Part model, mm, in its own coordinate system. Face numbers are marked on the shaded views. A direction names the side the tool comes from. Coordinates: 2 decimals unless noted, no trailing zeros. Loops run counter-clockwise (first coordinate to the right, second up) from the corner with the lowest first, then second, coordinate; pieces in that order, holes last.
```python
from build123d import *

# Parameters (mm, degrees)
BASPROSKE_W     = 20
BASPROSKE_H     = 48
TOOTHCUT_DEPTH  = 71.767224052
TEETHCUTS_COUNT = 22
TEETHCUTS_ANGLE = 343.636363636
BORSKE_R        = 10
BORE_DEPTH      = 50.0000508
KEYSKE_W        = 6
KEYSKE_H        = 12.8
KEYWAY_DEPTH    = 50.0000508


with BuildPart() as part:
    # BasProSke → Base-Revolve (revolve)
    with BuildSketch(Plane(origin=(0, 0, 0), x_dir=(1, 0, 0), z_dir=(0, 1, 0)), mode=Mode.PRIVATE) as base_revolve_sk:
        with Locations((10, 24)):
            Rectangle(BASPROSKE_W, BASPROSKE_H)
    revolve(base_revolve_sk.sketch.rotate(Axis((-10, 0, 0), (1, 0, 0)), 180), axis=Axis((-10, 0, 0), (1, 0, 0)))

    # TooCutSke → ToothCut (cut, through all)
    with BuildSketch(Plane(origin=(0, 0, 0), x_dir=(0, 0, -1), z_dir=(1, 0, 0))):
        with BuildLine():
            ThreePointArc((1.925610671, 38.951431611), (0, 38.999), (-1.925610671, 38.951431611))
            ThreePointArc((-1.925610671, 38.951431611), (-3.230295596, 43.579258947), (-5.738738554, 47.681295337))
            ThreePointArc((-5.738738554, 47.681295337), (0, 48.0254), (5.738738554, 47.681295337))
            ThreePointArc((5.738738554, 47.681295337), (3.230295596, 43.579258947), (1.925610671, 38.951431611))
        make_face()
    toothcut = extrude(amount=TOOTHCUT_DEPTH, mode=Mode.SUBTRACT)

    # TeethCuts: ToothCut ×22 about axis
    teethcuts_axis = Axis((-10, 0, 0), (1, 0, 0))
    for i in range(1, TEETHCUTS_COUNT):
        add(toothcut.rotate(teethcuts_axis, i * TEETHCUTS_ANGLE / (TEETHCUTS_COUNT - 1)), mode=Mode.SUBTRACT)

    # BorSke → Bore (cut, symmetric)
    with BuildSketch(Plane(origin=(0, 0, 0), x_dir=(0, 0, -1), z_dir=(1, 0, 0))):
        with Locations(Location((0, 0, 0), (0, 0, 180))):
            Circle(BORSKE_R)
    extrude(amount=BORE_DEPTH, both=True, mode=Mode.SUBTRACT)

    # KeySke → Keyway (cut, symmetric)
    with BuildSketch(Plane(origin=(0, 0, 0), x_dir=(0, 0, -1), z_dir=(1, 0, 0))):
        with Locations((0, 6.4)):
            Rectangle(KEYSKE_W, KEYSKE_H)
    extrude(amount=KEYWAY_DEPTH, both=True, mode=Mode.SUBTRACT)


solid = part.part
```
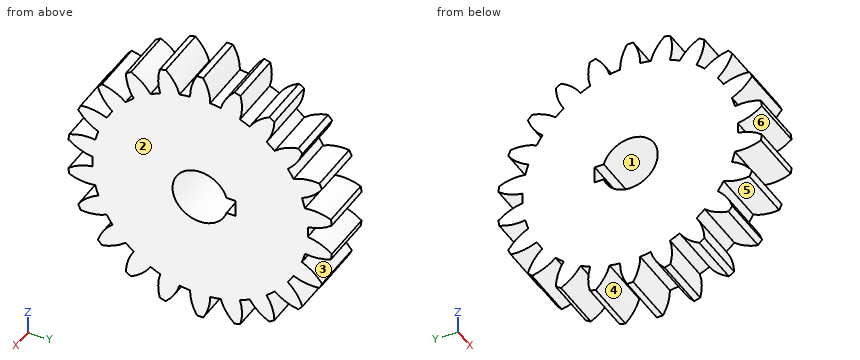
Q1. Saw through at A-A (y = 0). List the corners of the cut face in (x, z).
Q2. Saw through at C-C (y = -40.5). List the corners of the cut face in (x, z), plus the area to 3 significant figures.
Q3. Saw through at B-B (z = 0). List the corners of the cut face in (x, y).
Q4. Probe line 1 (Z direction, x = 13.75, y = 0); line 2 (Z direction, x = 17.25, y = -41.5); line 3 (Z direction, x = 11.5, y = 12.5). List the from-to ranges inside material, lowest first.
Q5. Mould opens along Y. For the marked faces 1, 2 and 3 say: released by +Y, released by -Y, zero draft, split by the parting line, or undercut.
Q6. Tool access for the marked faces 4, 5 and 6: list every direction of +Z, -Z, +X, -X, +Y, -Y with a clear straight run to the whole face (end or side of a thin tool).
Q7. Drop flat-ended pins along their axis: P1, Ø2, axis at x = 4.5, z = -11, coming from the +Y side; P2, Ø1, axis at x = 8, y = 11.5, coming from the -Z side; P3, Ø6.5, axis at x = 10, z = -1.5, coming from the -Y side. Give the stop position or say it passes through.
Q8. Saw through at D-D (z = 24). List the corners of the cut face in (x, y).
Checked values:
1. outline: (0, -48) - (20, -48) - (20, -10) - (0, -10) - close; (0, 10) - (20, 10) - (20, 48) - (0, 48) - close
2. outline: (0, -21.05) - (20, -21.05) - (20, -15.05) - (0, -15.05) - close; (0, -9.32) - (20, -9.32) - (20, -2.21) - (0, -2.21) - close; (0, 2.21) - (20, 2.21) - (20, 9.32) - (0, 9.32) - close; (0, 15.05) - (20, 15.05) - (20, 21.05) - (0, 21.05) - close
2. area: 524 mm2
3. outline: (0, -39) - (20, -39) - (20, -10) - (0, -10) - close; (0, 12.8) - (20, 12.8) - (20, 39) - (0, 39) - close
4. line 1: z = -48 to -10, 10 to 48
4. line 2: z = -21.06 to -15.9, -9.29 to -2.47, 2.47 to 9.29, 15.9 to 21.06
4. line 3: z = -46.34 to -3, 3 to 46.34
5. face 1: undercut
5. face 2: zero draft
5. face 3: released by +Y
6. face 4: -Z, +X, -X
6. face 5: +X, -X
6. face 6: +X, -X, -Y
7. P1: stops at y = 37.7
7. P2: stops at z = -45.94
7. P3: stops at y = -46.35
8. outline: (0, -33.11) - (20, -33.11) - (20, 33.11) - (0, 33.11) - close
